Autodesk Inventor part; units mm, degrees
ref_plane "YZ Plane" through (0, 0, 0) normal (1, 0, 0) x (0, 1, 0)
ref_plane "XZ Plane" through (0, 0, 0) normal (0, 1, 0) x (-1, 0, 0)
ref_plane "XY Plane" through (0, 0, 0) normal (0, 0, 1) x (1, 0, 0)
sketch "Sketch1" plane through (0, 0, 0) normal (0, 1, 0) x (-1, 0, 0)
  line L0 (-34, 24.5) -> (34, 24.5)
  line L1 (34, 24.5) -> (34, -24.5)
  line L2 (34, -24.5) -> (-34, -24.5)
  line L3 (-34, -24.5) -> (-34, 24.5)
  line L4 (-34, 24.5) -> (34, -24.5) construction
  line L5 (34, 24.5) -> (-34, -24.5) construction
  point P0 (0, 0)
  dimension "d0" = 49
  dimension "d1" = 68
extrude "Extrusion1" add sketch "Sketch1" along normal blind 2
sketch "Sketch3" plane through (0, 2, 0) normal (0, 1, 0) x (1, 0, 0)
  line L0 (-34, -24.5) -> (34, -24.5)
  line L1 (34, -24.5) -> (34, 24.5)
  arc A0 (34, -24.5) -> (34, -23.5) centre (33.818, -24) ccw
  point P0 (0, 0)
  dimension "d6" = 1
  dimension "d9" = 140
extrude "Extrusion2" add sketch "Sketch3" against normal blind 2
sketch "Sketch4" plane through (0, 2, 0) normal (0, 1, 0) x (1, 0, 0)
  line L0 (15, -8.9) -> (30, -8.9)
  line L1 (30, -8.9) -> (30, -20.5)
  line L2 (30, -20.5) -> (15, -20.5)
  line L3 (15, -20.5) -> (15, -8.9)
  line L4 (15, -8.9) -> (30, -20.5) construction
  line L5 (30, -8.9) -> (15, -20.5) construction
  line L6 (34, -23.5) -> (34, 24.5)
  line L7 (-34, -24.5) -> (34, -24.5)
  point P0 (0, 0)
  point P1 (22.5, -14.7)
  dimension "d12" = 15
  dimension "d13" = 11.6
  dimension "d14" = 4
  dimension "d15" = 4
extrude "Extrusion3" cut sketch "Sketch4" against normal blind 10
properties part number "side_lid_yes_hole_3DPrint"
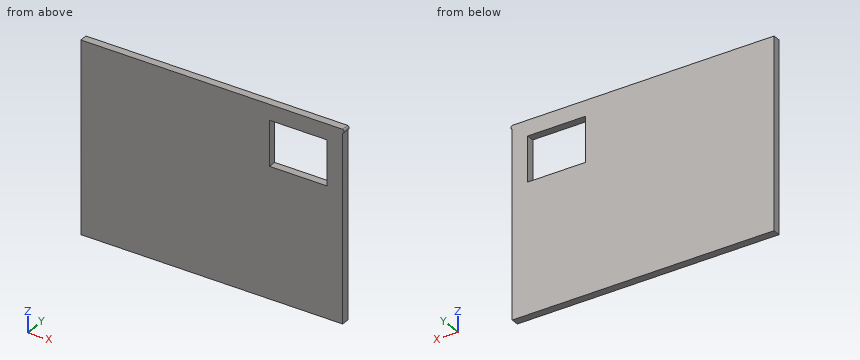
Check sheet for the modelled part. Datum: model origin and axes. Units: mm. Round coordinates to 2 decimals unless told otherwise and drop trailing zeros. Order: outer loops, then holes, each group sorted by start corner. A loop starts at its lowest first (then second) coordinate and runs counter-clockwise, first axis right, second up. Notation, with made-up numbers: M 54,-10 L 66,-10 A20 cw 66,0 Z; hole C 88,41.25 d10. An arc over 180 degrees is marked long. Answer in a Markdown table with one row per item.
(1) Gauge pin test, flat end, axial feed: pin 1 (0.6 mm diameter, centred on y = 1, z = 16.5, fed in from +X). Record the tip position at first contact, or that the pin passes through.
Findings:
| item | result |
|---|---|
| pin 1 | stops at x = 34 |
(2) Section check A-A on z = 12.5. Record the boundary of the cut face in (x, y), plus the area to 3 significant figures.
Findings:
| item | result |
|---|---|
| outline | M -34,0 L 15,0 L 15,2 L -34,2 Z; M 30,0 L 34,0 L 34,2 L 30,2 Z |
| area | 106 mm^2 |
(3) Section check B-B on y = 0.7. Record the boundary of the cut face in (x, z), plus the area to 3 significant figures.
Findings:
| item | result |
|---|---|
| outline | M -34,-24.5 L 34,-24.5 L 34,23.5 A0.53 ccw 34,24.5 L -34,24.5 Z; hole M 15,8.9 L 30,8.9 L 30,20.5 L 15,20.5 Z |
| area | 3,160 mm^2 |
(4) Section check C-C on x = 27.5. Record the boundary of the cut face in (y, z), plus the area to 3 significant figures.
Findings:
| item | result |
|---|---|
| outline | M 0,-24.5 L 2,-24.5 L 2,8.9 L 0,8.9 Z; M 0,20.5 L 2,20.5 L 2,24.5 L 0,24.5 Z |
| area | 74.8 mm^2 |
(5) Material ranges on line 1 along X through (y, z) = (0.95, 14); line 2 along Z through (x, y) = (17, 0.6); line 3 along X through (y, z) = (1.95, 0), recorded low to high. Write a range as from..to.
Findings:
| item | result |
|---|---|
| line 1 | x = -34..15, 30..34 |
| line 2 | z = -24.5..8.9, 20.5..24.5 |
| line 3 | x = -34..34 |
